```python
from build123d import *

# Parameters (mm, degrees)
SKETCH1_W           = 20
SKETCH1_H           = 10
BOSS_EXTRUDE1_DEPTH = 6.5
SKETCH2_W           = 20
SKETCH2_H           = 1.5
BOSS_EXTRUDE2_DEPTH = 4
SKETCH3_R           = 1.25
CUT_EXTRUDE1_DEPTH  = 15.941552797
SKETCH4_W           = 2
SKETCH4_H           = 6.5
BOSS_EXTRUDE3_DEPTH = 1.75
SKETCH5_W           = 3
SKETCH5_H           = 4
SKETCH5_W_2         = 3.3
CUT_EXTRUDE2_DEPTH  = 1.75


with BuildPart() as part:
    # Sketch1 → Boss-Extrude1 (new body)
    with BuildSketch(Plane(origin=(0, 0, 0), x_dir=(1, 0, 0), z_dir=(0, 1, 0))):
        Rectangle(SKETCH1_W, SKETCH1_H)
    extrude(amount=BOSS_EXTRUDE1_DEPTH)

    # Sketch2 → Boss-Extrude2 (add)
    with BuildSketch(Plane.XY.offset(5)):
        with Locations((0, 3.25)):
            Rectangle(SKETCH2_W, SKETCH2_H)
    extrude(amount=BOSS_EXTRUDE2_DEPTH)

    # Sketch3 → Cut-Extrude1 (cut, through all)
    with BuildSketch(Plane(origin=(0, 6.5, 0), x_dir=(1, 0, 0), z_dir=(0, 1, 0))):
        with Locations(Location((-5, -3, 0), (0, 0, 270))):
            Circle(SKETCH3_R)
        with Locations(Location((5, -3, 0), (0, 0, 270))):
            Circle(SKETCH3_R)
    extrude(amount=-CUT_EXTRUDE1_DEPTH, mode=Mode.SUBTRACT)

    # Sketch4 → Boss-Extrude3 (add)
    with BuildSketch(Plane(origin=(0, 0, -5), x_dir=(-1, 0, 0), z_dir=(0, 0, -1))):
        with Locations((3.5, 3.25)):
            Rectangle(SKETCH4_W, SKETCH4_H)
    extrude(amount=BOSS_EXTRUDE3_DEPTH)

    # Sketch5 → Cut-Extrude2 (cut)
    with BuildSketch(Plane(origin=(0, 4, 0), x_dir=(1, 0, 0), z_dir=(0, 1, 0))):
        with Locations((-4, -7)):
            Rectangle(SKETCH5_W, SKETCH5_H)
        with Locations((3.65, -7)):
            Rectangle(SKETCH5_W_2, SKETCH5_H)
    extrude(amount=-CUT_EXTRUDE2_DEPTH, mode=Mode.SUBTRACT)


solid = part.part
```
Model file for the job. Use its own axes, mm. A direction names the side the tool comes from. Round coordinates to 2 decimals unless told otherwise and drop trailing zeros. Write each loop counter-clockwise with the first axis right and the second up, starting at its lowest first coordinate (ties: lowest second). Pieces come first, ordered by that corner, then holes. Notation, with made-up numbers: (85.25, 10) - (135.25, 10) arc R4 cw to (135.25, 17) - close; hole circle Ø3 at (-40, 3.5). An arc over 180 degrees is marked (long way). One line per item, written item: value.
(1) Cut at D-D, the plane x = 0.5. Give the cut face in (y, z).
Values follow:
outline: (0, -5) - (6.5, -5) - (6.5, 5) - (4, 5) - (4, 9) - (2.5, 9) - (2.5, 5) - (0, 5) - close
(2) 3-axis set-ups, long thin cutter, end or side, ignore diameter. For faces 1 (the flat face through (8, 4, 7)), 2 (the flat face through (-4.5, 3, -6)), 3 (the flat face through (0, 2.5, 7)), 4 (the flat face through (8, 3, 9)), 5 (the flat face through (5.3, 3, 7)): which of +Z, -Z, +X, -X, +Y, -Y reach the whole face in a straight line?
Values follow:
face 1: +Z, +X, -X, +Y
face 2: -Z, -X, +Y, -Y
face 3: +Z, +X, -X, -Y
face 4: +Z, +X, -X, +Y, -Y
face 5: +Z, +Y, -Y
(3) Wall check: probe 1 along X at (y, z) = (3.5, 3); probe 2 along Z at (x, y) = (7, 0.75); probe 3 along Z at (x, y) = (-4.75, 6.25). Give the ranges that are in metal, low to high.
Values follow:
probe 1: x = -10 to -6.25, -3.75 to 3.75, 6.25 to 10
probe 2: z = -5 to 5
probe 3: z = -5 to 1.78, 4.22 to 5
(4) Two-plate mould, pull along X, no slides. Class faces 6 (the flat face through (8, 2.5, 7)), 7 (the flat face through (-10, 3, 1)), 8 (the flat face through (-5.5, 3, 7)), 9 (the flat face through (-2.5, 3, 7)): pulls with the +X half, pulls with the -X half, needs draft (parallel to the pull), parting line crosses it, or undercut.
Values follow:
face 6: needs draft
face 7: pulls with the -X half
face 8: undercut
face 9: undercut
(5) Drop flat-ended pins along their axis: P1, Ø0.5, axis at y = 2.5, z = -6, coming from the -X side; P2, Ø2, axis at x = 7.5, z = 8, coming from the +Y side; P3, Ø2, axis at x = 6.5, z = 6.5, coming from the -Y side; P4, Ø4, axis at x = 5, z = -3, coming from the -Y side. Give the stop position or say it passes through.
Values follow:
P1: stops at x = -4.5
P2: stops at y = 4
P3: stops at y = 2.5
P4: stops at y = 0
(6) Cut at B-B, the plane x = 5. Give the cut face in (y, z).
Values follow:
outline: (0, -5) - (6.5, -5) - (6.5, 1.75) - (0, 1.75) - close; (0, 4.25) - (6.5, 4.25) - (6.5, 5) - (0, 5) - close
(7) Cut at C-C, the plane y = 3.5. Give the cut face in (x, z).
Values follow:
outline: (-10, -5) - (-4.5, -5) - (-4.5, -6.75) - (-2.5, -6.75) - (-2.5, -5) - (10, -5) - (10, 9) - (5.3, 9) - (5.3, 5) - (2, 5) - (2, 9) - (-2.5, 9) - (-2.5, 5) - (-5.5, 5) - (-5.5, 9) - (-10, 9) - close; hole circle Ø2.5 at (-5, 3); hole circle Ø2.5 at (5, 3)
(8) Cut at A-A, the plane z = 3. Give the cut face in (x, y).
Values follow:
outline: (-10, 0) - (-6.25, 0) - (-6.25, 6.5) - (-10, 6.5) - close; (-3.75, 0) - (3.75, 0) - (3.75, 6.5) - (-3.75, 6.5) - close; (6.25, 0) - (10, 0) - (10, 6.5) - (6.25, 6.5) - close
